Source: three-view drawing plus pictorial views. Frame: mm from the lowest corner of the part. Coordinates: 2 decimals unless noted, no trailing zeros. Write each loop counter-clockwise with the first axis right and the second up, starting at its lowest first coordinate (ties: lowest second). Pieces come first, ordered by that corner, then holes. Notation, with made-up numbers: M 18,-30 L 41,-30 A17 cw 41,-26 Z; hole C 88.5,-17 d2. An arc over 180 degrees is marked long. Write item = value, one per line. Start each with the question number.
Item 1: First-contact query: pin 1 Ø3 at (x, z) = (4, 5.5) entering from -Y; pin 2 Ø1 at (x, z) = (2, 1) entering from +Y; pin 3 Ø3 at (y, z) = (6, 2.5) entering from -X; pin 4 Ø2 at (y, z) = (53.5, 8) entering from +X. Flat tips, straight axial feed; report the tip coordinate or a pass-through.
Item 2: Ray query, L1, parallel to Y at x = 9.25, z = 3.5; L2, parallel to Y at x = 5.5, z = 9; L3, parallel to X at y = 46, z = 4.75. Return the intervals inside material, ascending. Write a range as [from, to].
Item 3: Section A-A on y = 46. Output: boundary loops of the cut face in (x, z).
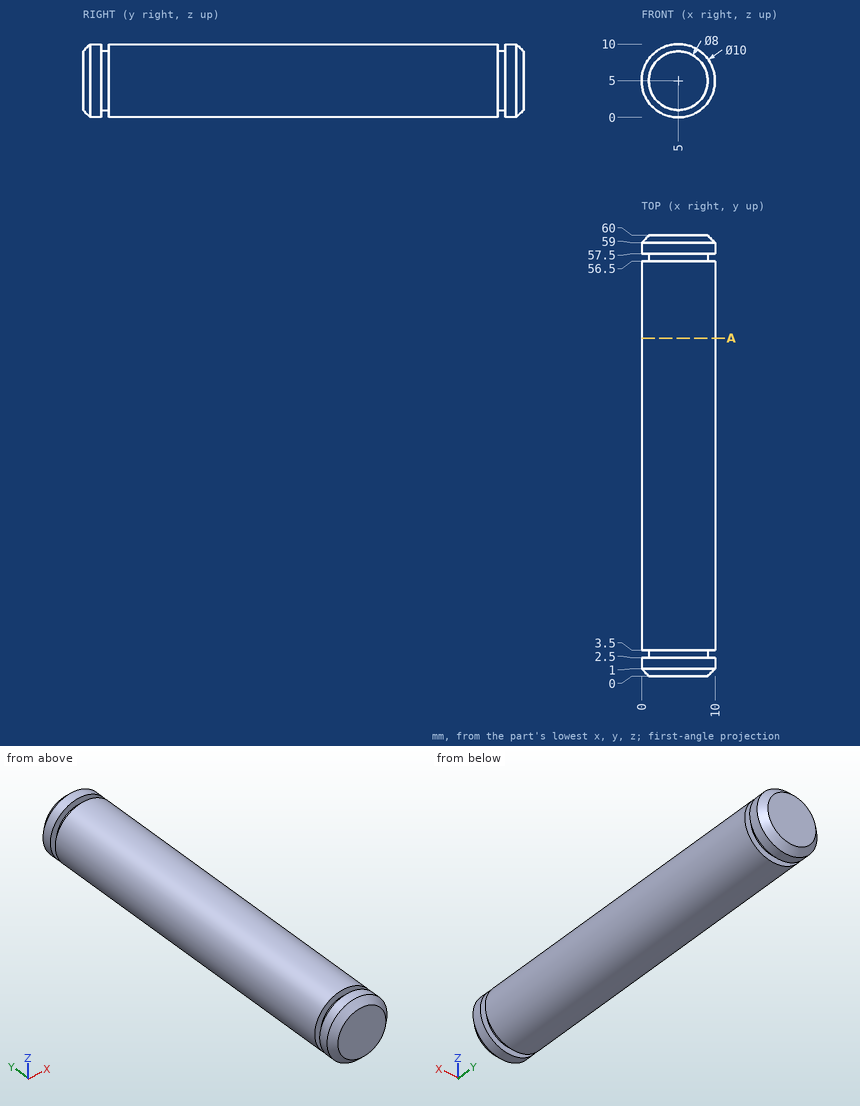
Responses:
q1.pin_1 = 0
q1.pin_2 = 59.5
q1.pin_3 = 0.1
q1.pin_4 = 9.58
q2.L1 = [0.51, 2.5], [3.5, 56.5], [57.5, 59.49]
q2.L2 = [0.03, 2.5], [3.5, 56.5], [57.5, 59.97]
q2.L3 = [0.01, 9.99]
q3.outline = C 5,5 d10
